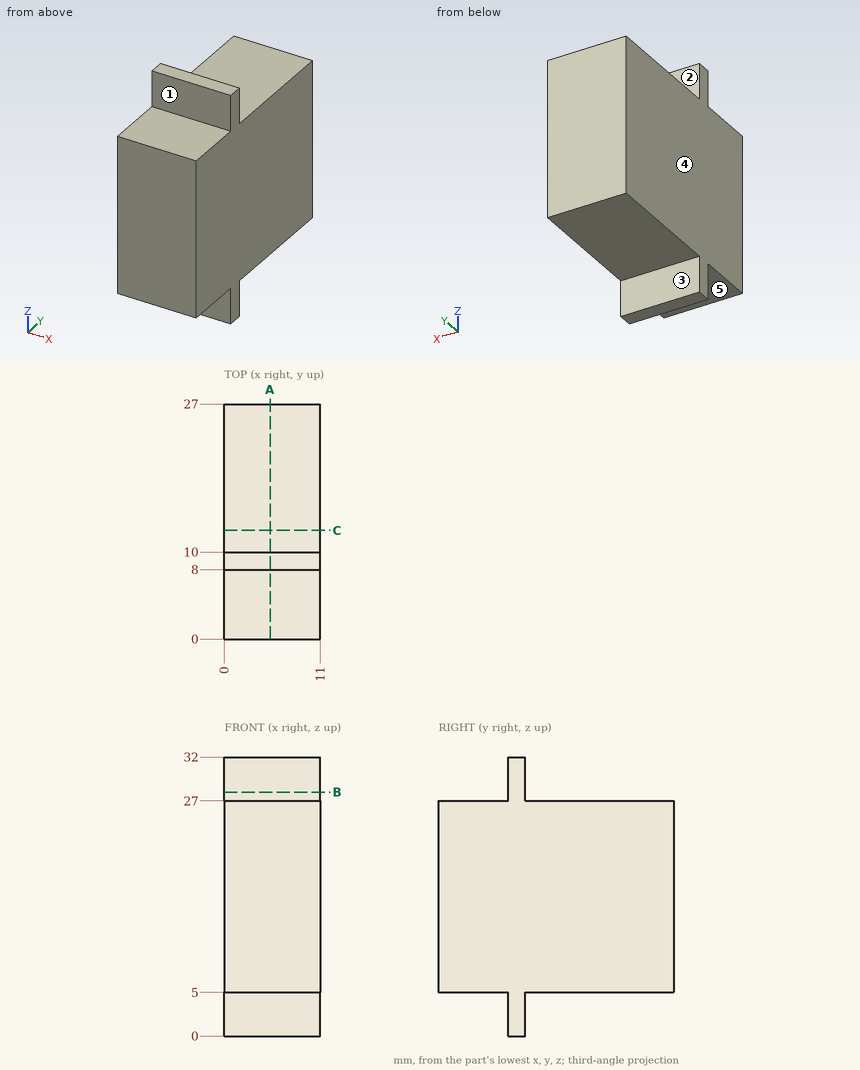
Verification items for this drawing (mm, ordinates from the low corner). A direction names the side the tool comes from. Round coordinates to 2 decimals unless told otherwise and drop trailing zeros. Write each loop counter-clockwise with the first axis right and the second up, starting at its lowest first coordinate (ties: lowest second). Pieces come first, ordered by that corner, then holes. Notation, with made-up numbers: (-6, -1) - (17, -1) arc R11 cw to (17, 6) - close; hole circle Ø9 at (3, 54). An arc over 180 degrees is marked (long way). Answer as a JSON object with one key per item and string values. Group by question number.
Q1. Tool access check on the marked faces 1, 2, 3, 4 and 5. Record the directions out of +Z, -Z, +X, -X, +Y, -Y that give a thin tool (end or side, any length) a straight path to the whole face; none if there is none.
Q2. Section check A-A, the plane x = 5.25. Enter the section's corners in (y, z), plus the area to 3 significant figures.
Q3. Go/stop test with flat-tipped pins: pin 1 Ø2.5 at (x, z) = (3, 2.5) entering from +Y; pin 2 Ø3 at (x, y) = (7.5, 16) entering from -Z; pin 3 Ø2.5 at (x, z) = (4, 3) entering from -Y. Record where each tip stops, or that it passes through.
Q4. Thickness scan on line 1 (Z direction, x = 4.25, y = 10.25). Record the ranges inside material, lowest first.
Q5. Section check C-C, the plane y = 12.5. Enter the section's corners in (x, z), plus the area to 3 significant figures.
Q6. Section check B-B, the plane z = 28. Enter the section's corners in (x, y), plus the area to 3 significant figures.
Found:
{
 "1": {"face 1": "+Z, +X, -X, -Y", "face 2": "+Z, +X, -X, +Y", "face 3": "-Z, +X, -X, +Y", "face 4": "+Z, -Z, -X, +Y, -Y", "face 5": "-Z, +X, -X, -Y"},
 "2": {"outline": "(0, 5) - (8, 5) - (8, 0) - (10, 0) - (10, 5) - (27, 5) - (27, 27) - (10, 27) - (10, 32) - (8, 32) - (8, 27) - (0, 27) - close", "area": "614 mm^2"},
 "3": {"pin 1": "stops at y = 10", "pin 2": "stops at z = 5", "pin 3": "stops at y = 8"},
 "4": {"line 1": "z = 5 to 27"},
 "5": {"outline": "(0, 5) - (11, 5) - (11, 27) - (0, 27) - close", "area": "242 mm^2"},
 "6": {"outline": "(0, 8) - (11, 8) - (11, 10) - (0, 10) - close", "area": "22.0 mm^2"}
}
